Here's how the part is built. I have some questions about the finished solid (model axes, mm). Face numbers are marked on the shaded views. Give positions to 0.01 mm unless a question says otherwise; leave off trailing zeros. Write each loop counter-clockwise with the first axis right and the second up, starting at its lowest first coordinate (ties: lowest second). Pieces come first, ordered by that corner, then holes. Notation, with made-up numbers: (13, 74.5) -> (70, 74.5) arc R26 cw to (70, 104.5) -> close; hole circle Ø10 at (75.5, -39). An arc over 180 degrees is marked (long way). Put each result on its own line as item: value. Start each with the question number.
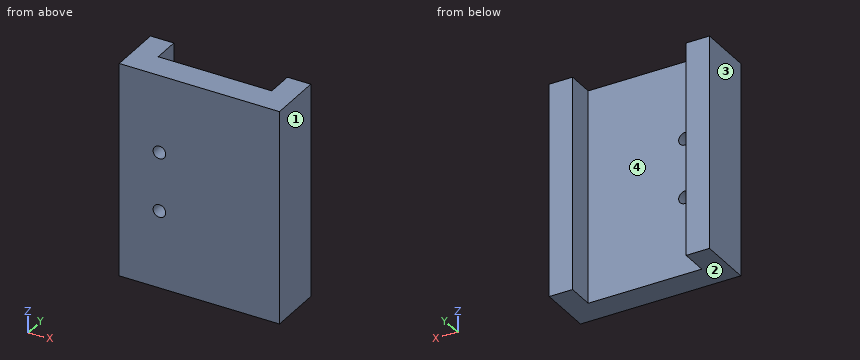
from build123d import *

# Parameters (mm, degrees)
SKETCH1_W           = 5.55
SKETCH1_H           = 6.35
SKETCH1_W_2         = 27
BOSS_EXTRUDE1_DEPTH = 50.8
SKETCH2_R           = 1.5
CUT_EXTRUDE1_DEPTH  = 56.72102386


with BuildPart() as part:
    # Sketch1 → Boss-Extrude1 (new body)
    with BuildSketch(Plane.XY):
        with Locations((-16.275, 9.525)):
            Rectangle(SKETCH1_W, SKETCH1_H)
        with Locations((-16.275, 3.175)):
            Rectangle(SKETCH1_W, SKETCH1_H)
        with Locations((0, 3.175)):
            Rectangle(SKETCH1_W_2, SKETCH1_H)
        with Locations((16.275, 9.525)):
            Rectangle(SKETCH1_W, SKETCH1_H)
        with Locations((16.275, 3.175)):
            Rectangle(SKETCH1_W, SKETCH1_H)
    extrude(amount=BOSS_EXTRUDE1_DEPTH)

    # Sketch2 → Cut-Extrude1 (cut, through all)
    with BuildSketch(Plane(origin=(0, 0, 0), x_dir=(1, 0, 0), z_dir=(0, 1, 0))):
        with Locations(Location((-9.5, -32.4, 0), (0, 0, 270))):
            Circle(SKETCH2_R)
        with Locations(Location((-9.5, -18.4, 0), (0, 0, 270))):
            Circle(SKETCH2_R)
    extrude(amount=CUT_EXTRUDE1_DEPTH, mode=Mode.SUBTRACT)


solid = part.part
1) I'm going to push a flat-ended pin straight in: pin 1 Ø10 at (x, z) = (-2, 7) entering from +Y. Where does the tip first touch, or does it pass through?
2) I want a section at B-B, the plane x = -9.5. Write out the boundary of the cut face in (y, z).
3) I want a section at C-C, the plane y = 9.25. Write out the boundary of the cut face in (x, z), and give its area (3 significant figures).
4) I want a section at D-D, the plane z = 20.5. Write out the boundary of the cut face in (x, y).
5) I want a section at A-A, the plane z = 32.4. Write out the boundary of the cut face in (x, y), and give its area (3 significant figures).
6) I need wall thicknesses on probe 1 along Z at (x, y) = (-9.5, 3.75); probe 2 along X at (y, z) = (9.5, 45); probe 3 along X at (y, z) = (3.25, 18.4). Which ranges of each line are inside material? Lowest first, please.
7) Thinking about a two-plate mould opening in X: for the marked faces 1, 2, 3 and 4, which applies, released by +X, released by -X, zero draft, split by the parting line, or undercut?
Established:
1. pin 1: stops at y = 6.35
2. outline: (0, 0) -> (6.35, 0) -> (6.35, 16.9) -> (0, 16.9) -> close; (0, 19.9) -> (6.35, 19.9) -> (6.35, 30.9) -> (0, 30.9) -> close; (0, 33.9) -> (6.35, 33.9) -> (6.35, 50.8) -> (0, 50.8) -> close
3. outline: (-19.05, 0) -> (-13.5, 0) -> (-13.5, 50.8) -> (-19.05, 50.8) -> close; (13.5, 0) -> (19.05, 0) -> (19.05, 50.8) -> (13.5, 50.8) -> close
3. area: 564 mm2
4. outline: (-19.05, 0) -> (19.05, 0) -> (19.05, 12.7) -> (13.5, 12.7) -> (13.5, 6.35) -> (-13.5, 6.35) -> (-13.5, 12.7) -> (-19.05, 12.7) -> close
5. outline: (-19.05, 0) -> (-11, 0) -> (-11, 6.35) -> (-13.5, 6.35) -> (-13.5, 12.7) -> (-19.05, 12.7) -> close; (-8, 0) -> (19.05, 0) -> (19.05, 12.7) -> (13.5, 12.7) -> (13.5, 6.35) -> (-8, 6.35) -> close
5. area: 293 mm2
6. probe 1: z = 0 to 16.9, 19.9 to 30.9, 33.9 to 50.8
6. probe 2: x = -19.05 to -13.5, 13.5 to 19.05
6. probe 3: x = -19.05 to -11, -8 to 19.05
7. face 1: released by +X
7. face 2: zero draft
7. face 3: released by -X
7. face 4: undercut
